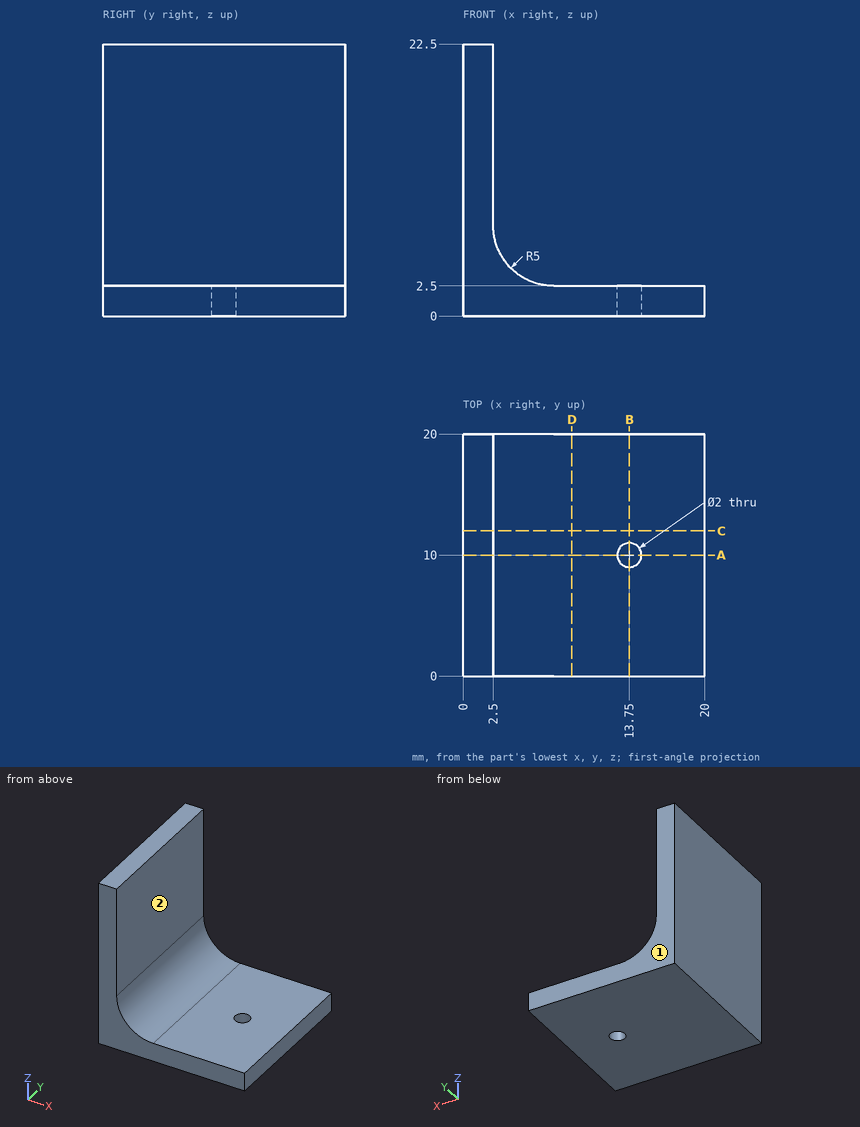
Study the drawing (mm; zero at the part's minimum x, y, z) and answer. A direction names the side the tool comes from. Give positions to 0.01 mm unless a question says otherwise; leave off trailing zeros. Order: outer loops, then holes, each group sorted by start corner. A loop starts at its lowest first (then second) coordinate and runs counter-clockwise, first axis right, second up. Notation, with made-up numbers: (-2.75, -36.75) - (43.25, -36.75) arc R6 ccw to (43.25, -32.75) - close; hole circle Ø11 at (10, 40). An arc over 180 degrees is marked (long way). Use one line per item in the form item = value. Start each with the question number.
(1) For the marked faces 1 and 2, determine the directions among +Z, -Z, +X, -X, +Y, -Y from which every point of the face is accessible in a straight line to the end or side of a thin tool.
(2) Consider line 1 (Y direction, x = 13.75, z = 1.1); line 2 (X direction, y = 11, z = 15.25). Determine where each line is inside the solid, lowest interval first. Write a range as from..to.
(3) A cutting plane is placed at C-C, the plane y = 12. Write down the section's boundary in (x, z), then the cut area to 3 significant figures.
(4) A cutting plane is placed at B-B, the plane x = 13.75. Write down the section's boundary in (y, z).
(5) Flat-ended cylindrical pins translate along their axes: pin 1 Ø10 at (x, y) = (10.5, 9.5) entering from +Z; pin 2 Ø3 at (y, z) = (11, 19.5) entering from +X; pin 3 Ø4 at (x, y) = (16, 11.5) entering from +Z. Find the tip coordinate at first contact, or state that the pin passes through.
(6) A cutting plane is placed at D-D, the plane x = 9. Write down the section's boundary in (y, z), then the cut area to 3 significant figures.
(7) A cutting plane is placed at A-A, the plane y = 10. Write down the section's boundary in (x, z).
Ans:
q1.face_1 = +Z, -Z, +X, -X, +Y
q1.face_2 = +Z, +X, +Y, -Y
q2.line_1 = 0..9, 11..20
q2.line_2 = 0..2.5
q3.outline = (0, 0) - (20, 0) - (20, 2.5) - (7.5, 2.5) arc R5 cw to (2.5, 7.5) - (2.5, 22.5) - (0, 22.5) - close
q3.area = 105 mm^2
q4.outline = (0, 0) - (9, 0) - (9, 2.5) - (0, 2.5) - close; (11, 0) - (20, 0) - (20, 2.5) - (11, 2.5) - close
q5.pin_1 = 2.92
q5.pin_2 = 2.5
q5.pin_3 = 2.5
q6.outline = (0, 0) - (20, 0) - (20, 2.5) - (0, 2.5) - close
q6.area = 50.0 mm^2
q7.outline = (0, 0) - (12.75, 0) - (12.75, 2.5) - (7.5, 2.5) arc R5 cw to (2.5, 7.5) - (2.5, 22.5) - (0, 22.5) - close; (14.75, 0) - (20, 0) - (20, 2.5) - (14.75, 2.5) - close
